Source: CAD feature listing. Evaluate the final solid. Frame: model axes, mm. Round coordinates to 2 decimals unless told otherwise and drop trailing zeros. Write each loop counter-clockwise with the first axis right and the second up, starting at its lowest first coordinate (ties: lowest second). Pieces come first, ordered by that corner, then holes.
from build123d import *

# Parameters (mm, degrees)
SKETCH1_R           = 4
SKETCH1_R_2         = 1.25
BOSS_EXTRUDE1_DEPTH = 2
FILLET1_R           = 1
CUT_EXTRUDE1_DEPTH  = 2


with BuildPart() as part:
    # Sketch1 → Boss-Extrude1 (new body)
    with BuildSketch(Plane(origin=(0, 0, 0), x_dir=(1, 0, 0), z_dir=(0, 1, 0))):
        with BuildLine():
            Line((987.5, 29.330127019), (952.858983849, 49.330127019))
            ThreePointArc((952.858983849, 49.330127019), (951.653079074, 49.829629131), (950.358983849, 50))
            Line((950.358983849, 50), (0, 50))
            Line((0, 50), (0, 0))
            Line((0, 0), (950.358983849, 0))
            ThreePointArc((950.358983849, 0), (951.653079074, 0.170370869), (952.858983849, 0.669872981))
            Line((952.858983849, 0.669872981), (987.5, 20.669872981))
            ThreePointArc((987.5, 20.669872981), (990, 25), (987.5, 29.330127019))
        make_face()
        with Locations((880, 25)):
            Circle(SKETCH1_R, mode=Mode.SUBTRACT)
        with Locations((10, 42)):
            Circle(SKETCH1_R_2, mode=Mode.SUBTRACT)
        with Locations((10, 8)):
            Circle(SKETCH1_R_2, mode=Mode.SUBTRACT)
    extrude(amount=BOSS_EXTRUDE1_DEPTH)

    # Fillet1
    fillet1_edges = [part.edges().sort_by_distance(p)[0] for p in [
        (0, 1, -50),
        (0, 1, 0),
    ]]
    fillet(fillet1_edges, radius=FILLET1_R)

    # Sketch2 → Cut-Extrude1 (cut)
    with BuildSketch(Plane(origin=(0, 2, 0), x_dir=(1, 0, 0), z_dir=(0, 1, 0))):
        with BuildLine():
            Line((8.184981615, 19.51366729), (0, 17.320508076))
            Line((0, 17.320508076), (0, 32.679491924))
            Line((0, 32.679491924), (8.184981615, 30.48633271))
            ThreePointArc((8.184981615, 30.48633271), (9.68136243, 30.549842721), (10.872908853, 31.457260037))
            ThreePointArc((10.872908853, 31.457260037), (31.180339887, 25), (10.872908853, 18.542739963))
            ThreePointArc((10.872908853, 18.542739963), (9.68136243, 19.450157279), (8.184981615, 19.51366729))
        make_face()
    extrude(amount=-CUT_EXTRUDE1_DEPTH, mode=Mode.SUBTRACT)


solid = part.part
1) Section query B-B on y = 0.7. Return the cut outline in (x, z).
Taken from the geometry:
outline: (0, -49) arc R1 ccw to (1, -50) - (950.36, -50) arc R5 ccw to (952.86, -49.33) - (987.5, -29.33) arc R5 ccw to (987.5, -20.67) - (952.86, -0.67) arc R5 ccw to (950.36, 0) - (1, 0) arc R1 ccw to (0, -1) - (0, -17.32) - (8.18, -19.51) arc R2.5 ccw to (10.87, -18.54) arc R11.18 cw (long way) to (10.87, -31.46) arc R2.5 ccw to (8.18, -30.49) - (0, -32.68) - close; hole circle Ø2.5 at (10, -42); hole circle Ø2.5 at (10, -8); hole circle Ø8 at (880, -25)
2) Contact query for a flat-ended pin moving along its axis: P1, Ø2, axis at x = 10, z = -8, coming from the +Y side. Output: stop coordinate, or through.
Taken from the geometry:
P1: passes through
3) Section query A-A on x = 20. Return the cut outline in (y, z).
Taken from the geometry:
outline: (0, -50) - (2, -50) - (2, -36.18) - (0, -36.18) - close; (0, -13.82) - (2, -13.82) - (2, 0) - (0, 0) - close
4) Pull-direction query (Z, two-part tool) for faces 1 (the face through (488, 2, -25)), 2 (the face through (31.173, 1.014, -25.395)), 3 (the face through (970.42, 0.99, -39.19)); classes: released by +Z, released by -Z, zero draft, split by the parting line, or undercut.
Taken from the geometry:
face 1: zero draft
face 2: undercut
face 3: released by -Z
5) Material intervals for line 1 (Z direction, x = 10, y = 1.1); line 2 (Z direction, x = 20, y = 0.9); line 3 (X direction, y = 0.6, z = -25), sorted ascending.
Taken from the geometry:
line 1: z = -50 to -43.25, -40.75 to -30.69, -19.31 to -9.25, -6.75 to 0
line 2: z = -50 to -36.18, -13.82 to 0
line 3: x = 31.18 to 876, 884 to 990
